Geometry check sheet. Reference: the model listing, model coordinates, mm. A direction names the side the tool comes from. Round coordinates to 2 decimals unless told otherwise and drop trailing zeros. Loops run counter-clockwise (first coordinate to the right, second up) from the corner with the lowest first, then second, coordinate; pieces in that order, holes last. Notation, with made-up numbers: (43, 18.25) - (80, 18.25) arc R34 ccw to (80, 55.25) - close; hole circle Ø11 at (-26, 45.25). An arc over 180 degrees is marked (long way). Answer as CSV lines item,"result". Start each with the question number.
1) Depth check by flat-ended pin: P1, Ø2, axis at x = -6, z = 14.5, coming from the +Y side; P2, Ø3, axis at x = 13, y = -8.5, coming from the -Z side; P3, Ø6, axis at x = -11, z = 8.5, coming from the -Y side. Enter the tip coordinate at first touch or a pass-through.
2) Access from +Z, -Z, +X, -X, +Y, -Y to the whole of each face (thin tool, end or side, straight path). Record for faces 1 (the cylindrical face through (-16.77, -16.233, 26.793)), 2 (the flat face through (-16, -17.5, 23)), 3 (the flat face through (4, 5, 5)).
3) Cross-section at B-B on x = 0. Record the boundary of the cut face in (y, z), and give its area (4 significant figures).
4) Cross-section at D-D on x = 15.5. Record the boundary of the cut face in (y, z), and give its area (3 significant figures).
5) Cross-section at A-A on z = 0. Record the boundary of the cut face in (x, y), and give its area (4 significant figures).
6) Cross-section at C-C on y = 1. Record the boundary of the cut face in (x, z), and give its area (3 significant figures).
7) Thickness scan on line 1 along Z through (x, y) = (0, -1.5); line 2 along Z through (x, y) = (0, 11); line 3 along Y through (x, z) = (11, 31). Record the ranges inside material, lowest first.
8) Draft check along X on faces 4 (the flat face through (15, 15, -15)), 5 (the flat face through (4, -5, 5)), 6 (the cylindrical face through (-28, 0, -21)). Enter one of: released by +X, released by -X, zero draft, split by the parting line, or undercut.
from build123d import *

# Parameters (mm, degrees)
F0_R     = 35
F0_R_2   = 20
F1_DEPTH = 15
F2_DEPTH = 5
F3_R     = 6.25
F4_DEPTH = 20
F5_R     = 3.686616
F6_DEPTH = 2.5


with BuildPart() as f1:
    # F0 (on Front) → F1 (new body, symmetric)
    with BuildSketch(Plane.XZ):
        Circle(F0_R)
        Circle(F0_R_2, mode=Mode.SUBTRACT)
    extrude(amount=F1_DEPTH, both=True)

    # F0 (on Front) → F2 (join, symmetric)
    with BuildSketch(Plane.XZ):
        Circle(F0_R_2)
    extrude(amount=F2_DEPTH, both=True)

    # F3 (on face) → F4 (cut, symmetric)
    with BuildSketch(Plane.XZ.offset(5)):
        Circle(F3_R)
    extrude(amount=F4_DEPTH, both=True, mode=Mode.SUBTRACT)

    # F5 (on face) → F6 (join)
    with BuildSketch(Plane.XZ.offset(15)):
        with Locations((-16.290108, 23.137607)):
            Circle(F5_R)
    extrude(amount=F6_DEPTH)


solid = f1.part
Answer block:
1,P1,"stops at y = 5"
1,P2,"stops at z = -33.06"
1,P3,"stops at y = -5"
2,face 1,"-Y"
2,face 2,"+Z, -Z, +X, -X, -Y"
2,face 3,"+Y"
3,outline,"(-15, -35) - (15, -35) - (15, -20) - (5, -20) - (5, -6.25) - (-5, -6.25) - (-5, -20) - (-15, -20) - close; (-15, 20) - (-5, 20) - (-5, 6.25) - (5, 6.25) - (5, 20) - (15, 20) - (15, 35) - (-15, 35) - close"
3,area,"1,175 mm^2"
4,outline,"(-15, -31.38) - (15, -31.38) - (15, -12.64) - (5, -12.64) - (5, 12.64) - (15, 12.64) - (15, 31.38) - (-15, 31.38) - (-15, 12.64) - (-5, 12.64) - (-5, -12.64) - (-15, -12.64) - close"
4,area,"1,380 mm^2"
5,outline,"(-35, -15) - (-20, -15) - (-20, -5) - (-6.25, -5) - (-6.25, 5) - (-20, 5) - (-20, 15) - (-35, 15) - close; (6.25, -5) - (20, -5) - (20, -15) - (35, -15) - (35, 15) - (20, 15) - (20, 5) - (6.25, 5) - close"
5,area,"1,175 mm^2"
6,outline,"circle Ø70 at (0, 0); hole circle Ø12.5 at (0, 0)"
6,area,"3,730 mm^2"
7,line 1,"z = -35 to -6.25, 6.25 to 35"
7,line 2,"z = -35 to -20, 20 to 35"
7,line 3,"y = -15 to 15"
8,face 4,"zero draft"
8,face 5,"undercut"
8,face 6,"split by the parting line"
